from build123d import *

# Parameters (mm, degrees)
SKETCH_1_R      = 2.5
SKETCH_1_R_2    = 2
SKETCH_1_R_3    = 1.5
EXTRUDE_1_DEPTH = 4
FILLET_1_R      = 5
CHAMFER_1_SIZE  = 0.5


with BuildPart() as part:
    # 草图1 → 凸台-拉伸1 (new body)
    with BuildSketch(Plane.XY):
        with BuildLine():
            Line((-27, 0), (-27, 70))
            Line((-27, 70), (-11.999997176, 70))
            Line((-11.999997176, 70), (22.879375353, 14.336463423))
            ThreePointArc((22.879375353, 14.336463423), (7.458447073, -25.949403987), (-27, 0))
        make_face()
        with Locations((0, 22.5)):
            Circle(SKETCH_1_R, mode=Mode.SUBTRACT)
        with Locations((22.5, 0)):
            Circle(SKETCH_1_R, mode=Mode.SUBTRACT)
        with Locations((0, -22.5)):
            Circle(SKETCH_1_R, mode=Mode.SUBTRACT)
        with Locations((-22.5, 0)):
            Circle(SKETCH_1_R, mode=Mode.SUBTRACT)
        with Locations((-22, 60)):
            Circle(SKETCH_1_R_2, mode=Mode.SUBTRACT)
        with Locations((-22, 50)):
            Circle(SKETCH_1_R_2, mode=Mode.SUBTRACT)
        with Locations((-22, 30)):
            Circle(SKETCH_1_R_2, mode=Mode.SUBTRACT)
        with Locations((-22, 40)):
            Circle(SKETCH_1_R_2, mode=Mode.SUBTRACT)
        with Locations((-12, 50)):
            Circle(SKETCH_1_R_2, mode=Mode.SUBTRACT)
        with Locations((0, 11)):
            Circle(SKETCH_1_R_3, mode=Mode.SUBTRACT)
        with Locations((11, 0)):
            Circle(SKETCH_1_R_3, mode=Mode.SUBTRACT)
        with Locations((0, -11)):
            Circle(SKETCH_1_R_3, mode=Mode.SUBTRACT)
        with Locations((-11, 0)):
            Circle(SKETCH_1_R_3, mode=Mode.SUBTRACT)
        with Locations((-12, 40)):
            Circle(SKETCH_1_R_2, mode=Mode.SUBTRACT)
        with Locations((-19, 14)):
            Circle(SKETCH_1_R, mode=Mode.SUBTRACT)
    extrude(amount=EXTRUDE_1_DEPTH)

    # 圆角1
    fillet_1_edges = [part.edges().sort_by_distance(p)[0] for p in [
        (-11.999997176, 70, 2),
    ]]
    fillet(fillet_1_edges, radius=FILLET_1_R)

    # 倒角1
    chamfer_1_edges = [part.edges().sort_by_distance(p)[0] for p in [
        (-27, 70, 2),
    ]]
    chamfer(chamfer_1_edges, length=CHAMFER_1_SIZE)


solid = part.part
The model under review builds one solid part; all positions refer to its coordinate system, in mm. Round coordinates to 2 decimals unless told otherwise and drop trailing zeros. Order: outer loops, then holes, each group sorted by start corner. A loop starts at its lowest first (then second) coordinate and runs counter-clockwise, first axis right, second up. Notation, with made-up numbers: (10, 84.25) -> (27, 84.25) arc R20 ccw to (27, 96.25) -> close; hole circle Ø9 at (46.5, 44). An arc over 180 degrees is marked (long way). Write item = value, one per line. Start each with the question number.
Item 1: Consider section B-B on y = 60. Write out the cut boundary in (x, z), plus the area to 3 significant figures.
Item 2: Consider section A-A on z = 0.95. Count the separate pieces of the cut face and the enclosed holes in it, plus the area to 3 significant figures.
Item 3: For line 1 along Y through (x, z) = (-12, 1.9); line 2 along X through (y, z) = (38.5, 2.4); line 3 along Y through (x, z) = (-13, 1.15), list the stretches that pass through material, from the lowest coordinate up.
Item 4: Mouldability with a two-part tool opening along X and no side actions: class faces 1 (the face through (-12.377, 69.392, 2.028)), 2 (the face through (8.128, -25.747, 1.972)), 3 (the face through (-22, 62, 2)) as released by +X, released by -X, zero draft, split by the parting line, or undercut.
Item 5: Consider section C-C on x = -18.5. Write out the cut boundary in (y, z).
Item 6: Consider section D-D on y = 50. Write out the cut boundary in (x, z), plus the area to 3 significant figures.
Item 7: Clearance check with flat-ended pins moving along their axes: pin 1 Ø4 at (x, y) = (0, -22.5) entering from +Z; pin 2 Ø3.5 at (x, y) = (11, 0) entering from +Z; pin 3 Ø1.5 at (x, z) = (13, 2) entering from +Y. State where each tip first meets the part, or that it passes through.
Conclusion:
q1.outline = (-27, 0) -> (-24, 0) -> (-24, 4) -> (-27, 4) -> close; (-20, 0) -> (-5.73, 0) -> (-5.73, 4) -> (-20, 4) -> close
q1.area = 69.1 mm2
q2.separate_pieces = 1
q2.enclosed_holes = 15
q2.area = 3,500 mm2
q3.line_1 = -24.19 to -1.12, 1.12 to 38, 42 to 48, 52 to 69.16
q3.line_2 = -27 to -23.32, -20.68 to -13.32, -10.68 to 7.74
q3.line_3 = -23.66 to 38.27, 41.73 to 48.27, 51.73 to 69.68
q4.face_1 = released by +X
q4.face_2 = split by the parting line
q4.face_3 = undercut
q5.outline = (-19.67, 0) -> (11.55, 0) -> (11.55, 4) -> (-19.67, 4) -> close; (16.45, 0) -> (70, 0) -> (70, 4) -> (16.45, 4) -> close
q6.outline = (-27, 0) -> (-24, 0) -> (-24, 4) -> (-27, 4) -> close; (-20, 0) -> (-14, 0) -> (-14, 4) -> (-20, 4) -> close; (-10, 0) -> (0.53, 0) -> (0.53, 4) -> (-10, 4) -> close
q6.area = 78.1 mm2
q7.pin_1 = through
q7.pin_2 = 4
q7.pin_3 = 31.3
